Build history of the part. All positions in model axes, mm. A direction names the side the tool comes from. Round coordinates to 2 decimals unless told otherwise and drop trailing zeros. Order: outer loops, then holes, each group sorted by start corner. A loop starts at its lowest first (then second) coordinate and runs counter-clockwise, first axis right, second up. Notation, with made-up numbers: M 73.25,23.5 L 113.25,23.5 A25 cw 113.25,35.5 Z; hole C -15,80.25 d1. An arc over 180 degrees is marked long. One line per question, with ' | ' between items. Start each with the question number.
Autodesk Inventor part; units mm, degrees
ref_plane "YZ Plane" through (0, 0, 0) normal (1, 0, 0) x (0, 1, 0)
ref_plane "XZ Plane" through (0, 0, 0) normal (0, 1, 0) x (-1, 0, 0)
ref_plane "XY Plane" through (0, 0, 0) normal (0, 0, 1) x (1, 0, 0)
sketch "Sketch1" plane through (0, 0, 0) normal (0, 0, 1) x (1, 0, 0)
  line L0 (0, 0) -> (37.5, 0)
  line L1 (37.5, 0) -> (37.5, 9)
  line L2 (37.5, 9) -> (0, 9)
  line L3 (0, 9) -> (0, 0)
  dimension "d0" = 37.5
  dimension "d1" = 9
extrude "Extrusion1" add sketch "Sketch1" along normal blind 5
sketch "Sketch2" plane through (37.5, 0, 0) normal (1, 0, 0) x (0, 0, -1)
  circle A0 centre (-2.5, 2.3541) radius 1.5
  circle A1 centre (-2.5, 5.3541) radius 1.5
  line L0 (0, 0) -> (-5, 0)
  line L1 (0, 9) -> (-5, 9)
  point P0 (-2.5, 0)
  dimension "d4" = 3
extrude "Extrusion2" add sketch "Sketch2" along normal blind 12
sketch "Sketch3" plane through (0, 0, 0) normal (-1, 0, 0) x (0, 0, 1)
  circle A0 centre (2.5, 7.5) radius 1.5
  circle A1 centre (2.5, 4.5) radius 1.5
  circle A2 centre (2.5, 1.5) radius 1.5
  line L0 (0, 9) -> (5, 9)
  line L1 (2.5, 7.5) -> (2.5, 9) construction
  line L2 (2.5, 1.5) -> (2.5, 0) construction
  line L3 (0, 0) -> (5, 0) construction
  dimension "d11" = 3
extrude "Extrusion3" add sketch "Sketch3" along normal blind 12
properties part number "ESC"
Item 1: Two-plate mould, pull along Y, no slides. Class faces 3 (the face through (-5.9, 4.5, 4)), 4 (the face through (18, 5, 0)), 5 (the face through (19, 9, 2)): +Y half, -Y half, draft (parallel to the pull), parting line (faces both ways), or undercut.
Item 2: Tool access for faces 1 (the face through (37.5, 4, 1)), 2 (the face through (-12, 8, 2)): list every direction of +Z, -Z, +X, -X, +Y, -Y with a clear straight run to the whole face (end or side of a thin tool).
Item 3: Flat gauge pin, fed straight in: pin 1 (3 mm diameter, centred on y = 5, z = 4.5, fed in from -X). Where does the tip first touch, or does it go through?
Item 4: Wall check: line 1 along X through (y, z) = (8.25, 4.4); line 2 along X through (y, z) = (6, 2.1); line 3 along Z through (x, y) = (-7.5, 1). Give the ranges that are in metal, low to high. Write a range as [from, to].
Item 5: Cut at B-B on z = 1.6. Write the cut outline in (x, y), then the cut area to 4 significant figures.
Item 6: Cut at C-C on y = 4.5. Write the cut outline in (x, z).
Results found:
1) face 3: undercut | face 4: draft | face 5: +Y half
2) face 1: +X | face 2: +Z, -Z, -X, +Y, -Y
3) pin 1: stops at x = -12
4) line 1: x = [0, 37.5] | line 2: x = [0, 49.5] | line 3: z = [1.09, 3.91]
5) outline: M -12,0.3 L 0,0.3 L 0,0 L 37.5,0 L 37.5,1.15 L 49.5,1.15 L 49.5,3.55 L 37.5,3.55 L 37.5,4.15 L 49.5,4.15 L 49.5,6.55 L 37.5,6.55 L 37.5,9 L 0,9 L 0,8.7 L -12,8.7 L -12,6.3 L 0,6.3 L 0,5.7 L -12,5.7 L -12,3.3 L 0,3.3 L 0,2.7 L -12,2.7 Z | area: 481.5 mm^2
6) outline: M -12,1 L 0,1 L 0,0 L 37.5,0 L 37.5,1.27 L 49.5,1.27 L 49.5,3.73 L 37.5,3.73 L 37.5,5 L 0,5 L 0,4 L -12,4 Z
